```python
from build123d import *

# Parameters (mm, degrees)
F1_DEPTH = 1


with BuildPart() as f1:
    # F0 (on Top) → F1 (new body)
    with BuildSketch(Plane.XY):
        with BuildLine():
            Line((-18.493242, 0.5), (-18.493242, -0.5))
            ThreePointArc((-18.493242, -0.5), (13.081475, -13.081475), (0.5, 18.493242))
            Line((0.5, 18.493242), (-0.5, 18.493242))
            ThreePointArc((-0.5, 18.493242), (-13.081475, 13.081475), (-18.493242, 0.5))
        make_face()
        with BuildLine():
            Line((-17.492856, -0.5), (-15.491933, -0.5))
            ThreePointArc((-15.491933, -0.5), (-10.960155, -10.960155), (-0.5, -15.491933))
            Line((-0.5, -15.491933), (-0.5, -17.492856))
            ThreePointArc((-0.5, -17.492856), (-12.374369, -12.374369), (-17.492856, -0.5))
        make_face(mode=Mode.SUBTRACT)
        with BuildLine():
            Line((-14.491377, -0.5), (-12.489996, -0.5))
            ThreePointArc((-12.489996, -0.5), (-8.838835, -8.838835), (-0.5, -12.489996))
            Line((-0.5, -12.489996), (-0.5, -14.491377))
            ThreePointArc((-0.5, -14.491377), (-10.253048, -10.253048), (-14.491377, -0.5))
        make_face(mode=Mode.SUBTRACT)
        with BuildLine():
            Line((-11.489125, -0.5), (-9.486833, -0.5))
            ThreePointArc((-9.486833, -0.5), (-6.717514, -6.717514), (-0.5, -9.486833))
            Line((-0.5, -9.486833), (-0.5, -11.489125))
            ThreePointArc((-0.5, -11.489125), (-8.131728, -8.131728), (-11.489125, -0.5))
        make_face(mode=Mode.SUBTRACT)
        with BuildLine():
            Line((-8.485281, -0.5), (-6.480741, -0.5))
            ThreePointArc((-6.480741, -0.5), (-4.596194, -4.596194), (-0.5, -6.480741))
            Line((-0.5, -6.480741), (-0.5, -8.485281))
            ThreePointArc((-0.5, -8.485281), (-6.010408, -6.010408), (-8.485281, -0.5))
        make_face(mode=Mode.SUBTRACT)
        with BuildLine():
            Line((-5.477226, -0.5), (-3.464102, -0.5))
            ThreePointArc((-3.464102, -0.5), (-2.474874, -2.474874), (-0.5, -3.464102))
            Line((-0.5, -3.464102), (-0.5, -5.477226))
            ThreePointArc((-0.5, -5.477226), (-3.889087, -3.889087), (-5.477226, -0.5))
        make_face(mode=Mode.SUBTRACT)
        with BuildLine():
            ThreePointArc((-0.5, -2.44949), (-1.767767, -1.767767), (-2.44949, -0.5))
            Line((-2.44949, -0.5), (-0.5, -0.5))
            Line((-0.5, -0.5), (-0.5, -2.44949))
        make_face(mode=Mode.SUBTRACT)
        with BuildLine():
            Line((15.491933, -0.5), (17.492856, -0.5))
            ThreePointArc((17.492856, -0.5), (12.374369, -12.374369), (0.5, -17.492856))
            Line((0.5, -17.492856), (0.5, -15.491933))
            ThreePointArc((0.5, -15.491933), (10.960155, -10.960155), (15.491933, -0.5))
        make_face(mode=Mode.SUBTRACT)
        with BuildLine():
            Line((12.489996, -0.5), (14.491377, -0.5))
            ThreePointArc((14.491377, -0.5), (10.253048, -10.253048), (0.5, -14.491377))
            Line((0.5, -14.491377), (0.5, -12.489996))
            ThreePointArc((0.5, -12.489996), (8.838835, -8.838835), (12.489996, -0.5))
        make_face(mode=Mode.SUBTRACT)
        with BuildLine():
            Line((9.486833, -0.5), (11.489125, -0.5))
            ThreePointArc((11.489125, -0.5), (8.131728, -8.131728), (0.5, -11.489125))
            Line((0.5, -11.489125), (0.5, -9.486833))
            ThreePointArc((0.5, -9.486833), (6.717514, -6.717514), (9.486833, -0.5))
        make_face(mode=Mode.SUBTRACT)
        with BuildLine():
            Line((6.480741, -0.5), (8.485281, -0.5))
            ThreePointArc((8.485281, -0.5), (6.010408, -6.010408), (0.5, -8.485281))
            Line((0.5, -8.485281), (0.5, -6.480741))
            ThreePointArc((0.5, -6.480741), (4.596194, -4.596194), (6.480741, -0.5))
        make_face(mode=Mode.SUBTRACT)
        with BuildLine():
            Line((3.464102, -0.5), (5.477226, -0.5))
            ThreePointArc((5.477226, -0.5), (3.889087, -3.889087), (0.5, -5.477226))
            Line((0.5, -5.477226), (0.5, -3.464102))
            ThreePointArc((0.5, -3.464102), (2.474874, -2.474874), (3.464102, -0.5))
        make_face(mode=Mode.SUBTRACT)
        with BuildLine():
            Line((0.5, -2.44949), (0.5, -0.5))
            Line((0.5, -0.5), (2.44949, -0.5))
            ThreePointArc((2.44949, -0.5), (1.767767, -1.767767), (0.5, -2.44949))
        make_face(mode=Mode.SUBTRACT)
        with BuildLine():
            Line((-0.5, 2.44949), (-0.5, 0.5))
            Line((-0.5, 0.5), (-2.44949, 0.5))
            ThreePointArc((-2.44949, 0.5), (-1.767767, 1.767767), (-0.5, 2.44949))
        make_face(mode=Mode.SUBTRACT)
        with BuildLine():
            Line((-3.464102, 0.5), (-5.477226, 0.5))
            ThreePointArc((-5.477226, 0.5), (-3.889087, 3.889087), (-0.5, 5.477226))
            Line((-0.5, 5.477226), (-0.5, 3.464102))
            ThreePointArc((-0.5, 3.464102), (-2.474874, 2.474874), (-3.464102, 0.5))
        make_face(mode=Mode.SUBTRACT)
        with BuildLine():
            Line((-6.480741, 0.5), (-8.485281, 0.5))
            ThreePointArc((-8.485281, 0.5), (-6.010408, 6.010408), (-0.5, 8.485281))
            Line((-0.5, 8.485281), (-0.5, 6.480741))
            ThreePointArc((-0.5, 6.480741), (-4.596194, 4.596194), (-6.480741, 0.5))
        make_face(mode=Mode.SUBTRACT)
        with BuildLine():
            Line((-9.486833, 0.5), (-11.489125, 0.5))
            ThreePointArc((-11.489125, 0.5), (-8.131728, 8.131728), (-0.5, 11.489125))
            Line((-0.5, 11.489125), (-0.5, 9.486833))
            ThreePointArc((-0.5, 9.486833), (-6.717514, 6.717514), (-9.486833, 0.5))
        make_face(mode=Mode.SUBTRACT)
        with BuildLine():
            Line((-12.489996, 0.5), (-14.491377, 0.5))
            ThreePointArc((-14.491377, 0.5), (-10.253048, 10.253048), (-0.5, 14.491377))
            Line((-0.5, 14.491377), (-0.5, 12.489996))
            ThreePointArc((-0.5, 12.489996), (-8.838835, 8.838835), (-12.489996, 0.5))
        make_face(mode=Mode.SUBTRACT)
        with BuildLine():
            Line((-15.491933, 0.5), (-17.492856, 0.5))
            ThreePointArc((-17.492856, 0.5), (-12.374369, 12.374369), (-0.5, 17.492856))
            Line((-0.5, 17.492856), (-0.5, 15.491933))
            ThreePointArc((-0.5, 15.491933), (-10.960155, 10.960155), (-15.491933, 0.5))
        make_face(mode=Mode.SUBTRACT)
        with BuildLine():
            Line((2.44949, 0.5), (0.5, 0.5))
            Line((0.5, 0.5), (0.5, 2.44949))
            ThreePointArc((0.5, 2.44949), (1.767767, 1.767767), (2.44949, 0.5))
        make_face(mode=Mode.SUBTRACT)
        with BuildLine():
            Line((5.477226, 0.5), (3.464102, 0.5))
            ThreePointArc((3.464102, 0.5), (2.474874, 2.474874), (0.5, 3.464102))
            Line((0.5, 3.464102), (0.5, 5.477226))
            ThreePointArc((0.5, 5.477226), (3.889087, 3.889087), (5.477226, 0.5))
        make_face(mode=Mode.SUBTRACT)
        with BuildLine():
            Line((8.485281, 0.5), (6.480741, 0.5))
            ThreePointArc((6.480741, 0.5), (4.596194, 4.596194), (0.5, 6.480741))
            Line((0.5, 6.480741), (0.5, 8.485281))
            ThreePointArc((0.5, 8.485281), (6.010408, 6.010408), (8.485281, 0.5))
        make_face(mode=Mode.SUBTRACT)
        with BuildLine():
            Line((11.489125, 0.5), (9.486833, 0.5))
            ThreePointArc((9.486833, 0.5), (6.717514, 6.717514), (0.5, 9.486833))
            Line((0.5, 9.486833), (0.5, 11.489125))
            ThreePointArc((0.5, 11.489125), (8.131728, 8.131728), (11.489125, 0.5))
        make_face(mode=Mode.SUBTRACT)
        with BuildLine():
            Line((14.491377, 0.5), (12.489996, 0.5))
            ThreePointArc((12.489996, 0.5), (8.838835, 8.838835), (0.5, 12.489996))
            Line((0.5, 12.489996), (0.5, 14.491377))
            ThreePointArc((0.5, 14.491377), (10.253048, 10.253048), (14.491377, 0.5))
        make_face(mode=Mode.SUBTRACT)
        with BuildLine():
            Line((0.5, 15.491933), (0.5, 17.492856))
            ThreePointArc((0.5, 17.492856), (12.374369, 12.374369), (17.492856, 0.5))
            Line((17.492856, 0.5), (15.491933, 0.5))
            ThreePointArc((15.491933, 0.5), (10.960155, 10.960155), (0.5, 15.491933))
        make_face(mode=Mode.SUBTRACT)
    extrude(amount=F1_DEPTH)


solid = f1.part
```
The listing builds one solid part. Answer for the finished solid, in the listing's coordinates (mm). Round coordinates to 2 decimals unless told otherwise and drop trailing zeros. Write each loop counter-clockwise with the first axis right and the second up, starting at its lowest first coordinate (ties: lowest second). Pieces come first, ordered by that corner, then holes. Notation, with made-up numbers: (80, 13) -> (127, 13) arc R24 ccw to (127, 51) -> close; hole circle Ø1 at (-19, 6). An arc over 180 degrees is marked (long way). Use CSV: the item, a comma, the result in double quotes. Start each with the question number.
(1) Section A-A on x = -11 is taken. Give the vertices of the cut face in (y, z), then the cut area to 3 significant figures.
(2) Section C-C on x = 12 is taken. Give the vertices of the cut face in (y, z).
(3) Consider L1, parallel to X at y = -16, z = 0.4; L2, parallel to X at y = 0, z = 0.45; L3, parallel to Y at x = 0, z = 0.3. Determine where each line is inside the solid, lowest interval first. Write a range as from..to.
(4) Section B-B on y = -15 is taken. Give the vertices of the cut face in (x, z), then the cut area to 3 significant figures.
(5) The mould has two halves that part along X. Classify faces 1 (the face through (0, 0, 1)), 2 (the face through (-13.5, -0.5, 0.5)): released by +X, released by -X, zero draft, split by the parting line, or undercut.
(6) Section D-D on z = 0.8 is taken. Count the separate pieces of the cut face and the enclosed holes in it, then the cut area to 3 significant figures.
(7) Each of these flat-tipped pins is pushed along its axis until it touches: pin 1 (0.5 mm diameter, centred on y = -17, z = 0.5, fed in from -X); pin 2 (0.5 mm diameter, centred on y = -14, z = 0.5, fed in from +X); pin 3 (0.5 mm diameter, centred on x = -10.5, z = 0.5, fed in from -Y). Where does it stop, or does it pass through?
A:
1,outline,"(-14.87, 0) -> (-13.61, 0) -> (-13.61, 1) -> (-14.87, 1) -> close; (-10.92, 0) -> (-9.45, 0) -> (-9.45, 1) -> (-10.92, 1) -> close; (-5.94, 0) -> (-3.35, 0) -> (-3.35, 1) -> (-5.94, 1) -> close; (-0.5, 0) -> (0.5, 0) -> (0.5, 1) -> (-0.5, 1) -> close; (3.35, 0) -> (5.94, 0) -> (5.94, 1) -> (3.35, 1) -> close; (9.45, 0) -> (10.92, 0) -> (10.92, 1) -> (9.45, 1) -> close; (13.61, 0) -> (14.87, 0) -> (14.87, 1) -> (13.61, 1) -> close"
1,area,"11.6 mm²"
2,outline,"(-14.08, 0) -> (-12.74, 0) -> (-12.74, 1) -> (-14.08, 1) -> close; (-9.81, 0) -> (-8.14, 0) -> (-8.14, 1) -> (-9.81, 1) -> close; (-3.5, 0) -> (3.5, 0) -> (3.5, 1) -> (-3.5, 1) -> close; (8.14, 0) -> (9.81, 0) -> (9.81, 1) -> (8.14, 1) -> close; (12.74, 0) -> (14.08, 0) -> (14.08, 1) -> (12.74, 1) -> close"
3,L1,"x = -9.29..-7.09, -0.5..0.5, 7.09..9.29"
3,L2,"x = -18.49..18.5"
3,L3,"y = -18.5..18.49"
4,outline,"(-10.83, 0) -> (-9.01, 0) -> (-9.01, 1) -> (-10.83, 1) -> close; (-3.91, 0) -> (3.91, 0) -> (3.91, 1) -> (-3.91, 1) -> close; (9.01, 0) -> (10.83, 0) -> (10.83, 1) -> (9.01, 1) -> close"
4,area,"11.4 mm²"
5,face 1,"zero draft"
5,face 2,"undercut"
6,separate pieces,"1"
6,enclosed holes,"24"
6,area,"445 mm²"
7,pin 1,"stops at x = -7.85"
7,pin 2,"stops at x = 12.38"
7,pin 3,"stops at y = -15.4"
